```python
from build123d import *

# Parameters (mm, degrees)
EXTRUDE_1_DEPTH                 = 60
FILLET_1_R                      = 10
CUT_EXTRUDE_1_DEPTH             = 93.054331955
CUT_EXTRUDE_1_DEPTH_BACK        = 93.054331955
SKETCH_2_R                      = 6.25
CUT_EXTRUDE_2_DEPTH             = 93.054331955
CUT_EXTRUDE_2_DEPTH_BACK        = 93.054331955
SKETCH_3_R                      = 19.5
CUT_EXTRUDE_3_DEPTH             = 2
MM_1_D                          = 8
MM_1_DEPTH                      = 6
MM_1_TIP                        = 2.403442476
CUT_EXTRUDE_4_REACH             = 120.41
CUT_EXTRUDE_4_END_RADIUS        = 19.5
SKETCH_9_R                      = 7
CUT_EXTRUDE_4_DIRECTION_2_DEPTH = 119.410303775
CUT_EXTRUDE_5_REACH             = 120.41
SKETCH_10_R                     = 9
HOLE_WIZARD_M8_2_AT_2_COUNT     = 2
HOLE_WIZARD_M8_2_AT_2_PITCH     = 25.455844123
HOLE_WIZARD_M8_2_AT_3_COUNT     = 2
HOLE_WIZARD_M8_2_AT_3_PITCH     = 36
HOLE_WIZARD_M8_2_AT_4_COUNT     = 2
HOLE_WIZARD_M8_2_AT_4_PITCH     = 25.455844123


with BuildPart() as part:
    # 草图1 → 凸台-拉伸1 (new body)
    with BuildSketch(Plane(origin=(0, 0, 0), x_dir=(1, 0, 0), z_dir=(0, 1, 0))):
        with BuildLine():
            ThreePointArc((-38.5, 16.5), (-35.796358171, 30.672887556), (-28.065156277, 42.855208274))
            ThreePointArc((-28.065156277, 42.855208274), (-38.480773302, 39.852739934), (-43, 30))
            Line((-43, 30), (-43, -30))
            ThreePointArc((-43, -30), (-38.480773302, -39.852739934), (-28.065156277, -42.855208274))
            ThreePointArc((-28.065156277, -42.855208274), (-35.796358171, -30.672887556), (-38.5, -16.5))
            Line((-38.5, -16.5), (-38.5, 16.5))
        make_face()
        with BuildLine():
            ThreePointArc((-17, 30), (-20.147260066, 38.480773302), (-28.065156277, 42.855208274))
            ThreePointArc((-28.065156277, 42.855208274), (-35.796358171, 30.672887556), (-38.5, 16.5))
            Line((-38.5, 16.5), (-38.5, -16.5))
            ThreePointArc((-38.5, -16.5), (-35.796358171, -30.672887556), (-28.065156277, -42.855208274))
            ThreePointArc((-28.065156277, -42.855208274), (-20.147260066, -38.480773302), (-17, -30))
            Line((-17, -30), (-17, 30))
        make_face()
        with BuildLine():
            ThreePointArc((17, 30), (20.147260066, 38.480773302), (28.065156277, 42.855208274))
            ThreePointArc((28.065156277, 42.855208274), (0, 55), (-28.065156277, 42.855208274))
            ThreePointArc((-28.065156277, 42.855208274), (-20.147260066, 38.480773302), (-17, 30))
            Line((-17, 30), (-17, -30))
            ThreePointArc((-17, -30), (-20.147260066, -38.480773302), (-28.065156277, -42.855208274))
            ThreePointArc((-28.065156277, -42.855208274), (0, -55), (28.065156277, -42.855208274))
            ThreePointArc((28.065156277, -42.855208274), (20.147260066, -38.480773302), (17, -30))
            Line((17, -30), (17, 30))
        make_face()
        with BuildLine():
            Line((38.5, -16.5), (38.5, 16.5))
            ThreePointArc((38.5, 16.5), (35.796358171, 30.672887556), (28.065156277, 42.855208274))
            ThreePointArc((28.065156277, 42.855208274), (20.147260066, 38.480773302), (17, 30))
            Line((17, 30), (17, -30))
            ThreePointArc((17, -30), (20.147260066, -38.480773302), (28.065156277, -42.855208274))
            ThreePointArc((28.065156277, -42.855208274), (35.796358171, -30.672887556), (38.5, -16.5))
        make_face()
        with BuildLine():
            ThreePointArc((28.065156277, 42.855208274), (35.796358171, 30.672887556), (38.5, 16.5))
            Line((38.5, 16.5), (38.5, -16.5))
            ThreePointArc((38.5, -16.5), (35.796358171, -30.672887556), (28.065156277, -42.855208274))
            ThreePointArc((28.065156277, -42.855208274), (38.480773302, -39.852739934), (43, -30))
            Line((43, -30), (43, 30))
            ThreePointArc((43, 30), (38.480773302, 39.852739934), (28.065156277, 42.855208274))
        make_face()
    extrude(amount=EXTRUDE_1_DEPTH)

    # 圆角1
    fillet_1_edges = [part.edges().sort_by_distance(p)[0] for p in [
        (-28.065156277, 30, 42.855208274),
        (-28.065156277, 30, -42.855208274),
        (28.065156277, 30, -42.855208274),
        (28.065156277, 30, 42.855208274),
    ]]
    fillet(fillet_1_edges, radius=FILLET_1_R)

    # 草图2 → 切除-拉伸1 (cut, two sides: drawn at the far end of the back side and taken through both)
    with BuildSketch(Plane(origin=(0, 60, 0), x_dir=(1, 0, 0), z_dir=(0, 1, 0)).offset(-CUT_EXTRUDE_1_DEPTH_BACK)):
        with Locations(Location((-30, 30, 0), (0, 0, 270))):
            Circle(SKETCH_2_R)
        with Locations(Location((30, 30, 0), (0, 0, 270))):
            Circle(SKETCH_2_R)
        with Locations(Location((30, -30, 0), (0, 0, 270))):
            Circle(SKETCH_2_R)
        with Locations(Location((-30, -30, 0), (0, 0, 270))):
            Circle(SKETCH_2_R)
    extrude(amount=CUT_EXTRUDE_1_DEPTH + CUT_EXTRUDE_1_DEPTH_BACK, mode=Mode.SUBTRACT)

    # 草图3 → 切除-拉伸2 (cut, two sides: drawn at the far end of the back side and taken through both)
    with BuildSketch(Plane(origin=(0, 60, 0), x_dir=(1, 0, 0), z_dir=(0, 1, 0)).offset(-CUT_EXTRUDE_2_DEPTH_BACK)):
        with Locations((0, 16.5)):
            Circle(SKETCH_3_R)
        with Locations((0, -16.5)):
            Circle(SKETCH_3_R)
        Circle(SKETCH_3_R)
    extrude(amount=CUT_EXTRUDE_2_DEPTH + CUT_EXTRUDE_2_DEPTH_BACK, mode=Mode.SUBTRACT)

    # 草图4 → 切除-拉伸3 (cut)
    with BuildSketch(Plane(origin=(0, 60, 0), x_dir=(1, 0, 0), z_dir=(0, 1, 0))):
        with BuildLine():
            Line((25, 16.5), (25, -16.5))
            ThreePointArc((25, -16.5), (0, -41.5), (-25, -16.5))
            Line((-25, -16.5), (-25, 16.5))
            ThreePointArc((-25, 16.5), (0, 41.5), (25, 16.5))
        make_face()
        with BuildLine():
            Line((21, 16.5), (21, -16.5))
            ThreePointArc((21, -16.5), (0, -37.5), (-21, -16.5))
            Line((-21, -16.5), (-21, 16.5))
            ThreePointArc((-21, 16.5), (0, 37.5), (21, 16.5))
        make_face(mode=Mode.SUBTRACT)
    cut_extrude_3 = extrude(amount=-CUT_EXTRUDE_3_DEPTH, mode=Mode.SUBTRACT)

    # 镜向1: 切除-拉伸3 across plane
    add(cut_extrude_3.mirror(Plane.ZX.offset(30)), mode=Mode.SUBTRACT)

    # 大小mm 暗销孔1
    with Locations(Plane(origin=(0, 60, -47.035270406), x_dir=(0, 0, 1), z_dir=(0, 1, 0))):
        with Locations((0, 0), (95, 0)):
            Hole(MM_1_D / 2, depth=MM_1_DEPTH)
            with Locations((0, 0, -(MM_1_DEPTH + MM_1_TIP / 2))):  # 118° drill point
                Cone(0, MM_1_D / 2, MM_1_TIP, mode=Mode.SUBTRACT)

    # 切除-拉伸4: up to this cylinder (the profile starts outside it)
    cut_extrude_4_end = Plane(origin=(0, 30, 0), z_dir=(0, 1, 0)) * Cylinder(CUT_EXTRUDE_4_END_RADIUS, 280.82, mode=Mode.PRIVATE)
    # 草图9 → 切除-拉伸4 (cut, up to the surface)
    with BuildSketch(Plane(origin=(43, 0, 0), x_dir=(0, 0, -1), z_dir=(1, 0, 0)), mode=Mode.PRIVATE) as cut_extrude_4_sk1:
        with Locations(Location((0, 30, 0), (0, 0, 180))):
            Circle(SKETCH_9_R)
    cut_extrude_4_tool1 = extrude(cut_extrude_4_sk1.sketch, amount=-CUT_EXTRUDE_4_REACH, mode=Mode.PRIVATE) - cut_extrude_4_end
    add(cut_extrude_4_tool1.solids().sort_by_distance((43, 30, 0))[0], mode=Mode.SUBTRACT)

    # 草图9 → 切除-拉伸4 direction 2 (cut)
    with BuildSketch(Plane(origin=(43, 0, 0), x_dir=(0, 0, -1), z_dir=(1, 0, 0))):
        with Locations(Location((0, 30, 0), (0, 0, 180))):
            Circle(SKETCH_9_R)
    extrude(amount=CUT_EXTRUDE_4_DIRECTION_2_DEPTH, mode=Mode.SUBTRACT)

    # 草图10 → 切除-拉伸5 (cut, up to next)
    with BuildSketch(Plane.ZY.offset(43), mode=Mode.PRIVATE) as cut_extrude_5_sk1:
        with Locations((0, 30)):
            Circle(SKETCH_10_R)
    cut_extrude_5_tool1 = extrude(cut_extrude_5_sk1.sketch, amount=-CUT_EXTRUDE_5_REACH, mode=Mode.PRIVATE) & part.part
    add(cut_extrude_5_tool1.solids().sort_by_distance((-43, 30, 0))[0], mode=Mode.SUBTRACT)

    # 草图13 → M8 螺纹孔2 (revolve, cut)
    with BuildSketch(Plane(origin=(43, 48, 0), x_dir=(0, 0, -1), z_dir=(0, 1, 0))):
        Polygon((0, 0), (0, 17.042926105), (3.4, 15), (3.4, 0), align=None)
    hole_wizard_m8_2 = revolve(axis=Axis((49.35, 48, 0), (-1, 0, 0)), mode=Mode.SUBTRACT)

    # M8 螺纹孔2 at 2: M8 螺纹孔2 ×2
    with Locations(*[Vector(0, -0.7071067811865476, -0.7071067811865476) * (i * HOLE_WIZARD_M8_2_AT_2_PITCH) for i in range(1, HOLE_WIZARD_M8_2_AT_2_COUNT)]):
        add(hole_wizard_m8_2, mode=Mode.SUBTRACT)

    # M8 螺纹孔2 at 3: M8 螺纹孔2 ×2
    with Locations(*[(0, -i * HOLE_WIZARD_M8_2_AT_3_PITCH, 0) for i in range(1, HOLE_WIZARD_M8_2_AT_3_COUNT)]):
        add(hole_wizard_m8_2, mode=Mode.SUBTRACT)

    # M8 螺纹孔2 at 4: M8 螺纹孔2 ×2
    with Locations(*[Vector(0, -0.7071067811865475, 0.7071067811865476) * (i * HOLE_WIZARD_M8_2_AT_4_PITCH) for i in range(1, HOLE_WIZARD_M8_2_AT_4_COUNT)]):
        add(hole_wizard_m8_2, mode=Mode.SUBTRACT)

    # 镜向2: M8 螺纹孔2 across plane
    add(hole_wizard_m8_2.mirror(Plane(origin=(0, 0, 0), x_dir=(0, 0, 1), z_dir=(1, 0, 0))), mode=Mode.SUBTRACT)

    # 镜向2 copy 1 sketch → 镜向2 copy 1 (revolve, cut)
    with BuildSketch(Plane(origin=(-43, 30, -18), x_dir=(0, 0, -1), z_dir=(0, 1, 0))):
        Polygon((0, 0), (0, -17.042926105), (3.4, -15), (3.4, 0), align=None)
    revolve(axis=Axis((-49.35, 30, -18), (-1, 0, 0)), mode=Mode.SUBTRACT)

    # 镜向2 copy 2 sketch → 镜向2 copy 2 (revolve, cut)
    with BuildSketch(Plane(origin=(-43, 12, 0), x_dir=(0, 0, -1), z_dir=(0, 1, 0))):
        Polygon((0, 0), (0, -17.042926105), (3.4, -15), (3.4, 0), align=None)
    revolve(axis=Axis((-49.35, 12, 0), (-1, 0, 0)), mode=Mode.SUBTRACT)

    # 镜向2 copy 3 sketch → 镜向2 copy 3 (revolve, cut)
    with BuildSketch(Plane(origin=(-43, 30, 18), x_dir=(0, 0, -1), z_dir=(0, 1, 0))):
        Polygon((0, 0), (0, -17.042926105), (3.4, -15), (3.4, 0), align=None)
    revolve(axis=Axis((-49.35, 30, 18), (-1, 0, 0)), mode=Mode.SUBTRACT)


solid = part.part
```
For this review, take the finished solid that the model builds, in its own axes (mm). A direction names the side the tool comes from. Give positions to 0.01 mm unless a question says otherwise; leave off trailing zeros. Order: outer loops, then holes, each group sorted by start corner. A loop starts at its lowest first (then second) coordinate and runs counter-clockwise, first axis right, second up.
1) For faces 5 (the face through (35.605, 28.979, 14.757)), 6 (the face through (-0.462, 59.014, -37.495)), 7 (the face through (19.396, 22.913, 2.009)), 8 (the face through (-30.512, 32.703, 8.584)), list the 3-axis set-ups (+Z, -Z, +X, -X, +Y, -Y) from which the entire face can be reached by the end or side of a thin tool; tool diameter is ignored.
2) The part is to be moulded in two halves that separate along Y. For faces 1 (the face through (28, 60, -1)), 2 (the face through (-1.53, 56.96, 44.27)), 3 (the face through (22, 2, 3)), 4 (the face through (-35.6, 29.9, 21.4)), say which applies: released by +Y, released by -Y, zero draft, split by the parting line, or undercut.
3) Wall thickness on line 1 (Y direction, x = 37, z = 0); line 2 (Z direction, x = -35.5, y = 32); line 3 (Z direction, x = -30, y = 14): over which ranges is each line inside the solid? List them lowest first.
4) Take a section at B-B (y = 28). State how many separate pieces and enclosed holes the cut face has, then the cut area to 3 significant figures.
5) Take a section at A-A (x = -34.5). Give the boundary of the cut face in (y, z).
6) Take a section at C-C (x = -7). Give the boundary of the cut face in (y, z), then the cut area to 3 significant figures.
7) Insertion check: pin 1 (2 mm diameter, centred on x = 17, y = 47, fed in from +Z); pin 2 (23.5 mm diameter, centred on x = 0, z = -16.5, fed in from +Y); pin 3 (3 mm diameter, centred on y = 10.5, z = 36, fed in from +X); pin 4 (5 mm diameter, centred on x = 0, z = 47.96, fed in from +Y). Each pin has a flat end and moves straight along its axis. Give the tip position at first contact, or say it passes through.
Derived:
1. face 5: +X
1. face 6: +Y
1. face 7: +Y, -Y
1. face 8: -X
2. face 1: released by +Y
2. face 2: zero draft
2. face 3: released by -Y
2. face 4: undercut
3. line 1: y = 0 to 8.6, 15.4 to 23, 37 to 44.6, 51.4 to 60
3. line 2: z = -41.78 to -32.97, -27.03 to -20.75, -15.25 to -8.77, 8.77 to 15.25, 20.75 to 27.03, 32.97 to 41.78
3. line 3: z = -43.12 to -36.25, -23.75 to -2.75, 2.75 to 23.75, 36.25 to 43.12
4. separate pieces: 2
4. enclosed holes: 4
4. area: 4,160 mm2
5. outline: (0, -42.2) - (60, -42.2) - (60, -34.34) - (0, -34.34) - close; (0, -25.66) - (60, -25.66) - (60, 25.66) - (0, 25.66) - close; (0, 34.34) - (60, 34.34) - (60, 42.2) - (0, 42.2) - close; hole circle Ø6.8 at (12, 0); hole circle Ø18 at (30, 0); hole circle Ø6.8 at (30, -18); hole circle Ø6.8 at (30, 18); hole circle Ø6.8 at (48, 0)
6. outline: (0, -54.36) - (60, -54.36) - (60, -40.5) - (58, -40.5) - (58, -36.3) - (60, -36.3) - (60, -34.7) - (0, -34.7) - (0, -36.3) - (2, -36.3) - (2, -40.5) - (0, -40.5) - close; (0, 34.7) - (60, 34.7) - (60, 36.3) - (58, 36.3) - (58, 40.5) - (60, 40.5) - (60, 54.36) - (0, 54.36) - (0, 40.5) - (2, 40.5) - (2, 36.3) - (0, 36.3) - close
6. area: 2,330 mm2
7. pin 1: stops at z = 51.52
7. pin 2: passes through
7. pin 3: stops at x = 42.2
7. pin 4: stops at y = 53.1
